Verification items for this drawing (mm, ordinates from the low corner). A direction names the side the tool comes from. Coordinates: 2 decimals unless noted, no trailing zeros. Order: outer loops, then holes, each group sorted by start corner. A loop starts at its lowest first (then second) coordinate and runs counter-clockwise, first axis right, second up. Notation, with made-up numbers: M 61,47.5 L 72,47.5 A20 ccw 72,68.5 Z; hole C 37,25.25 d10. An arc over 180 degrees is marked long. Write item = value, one per line.
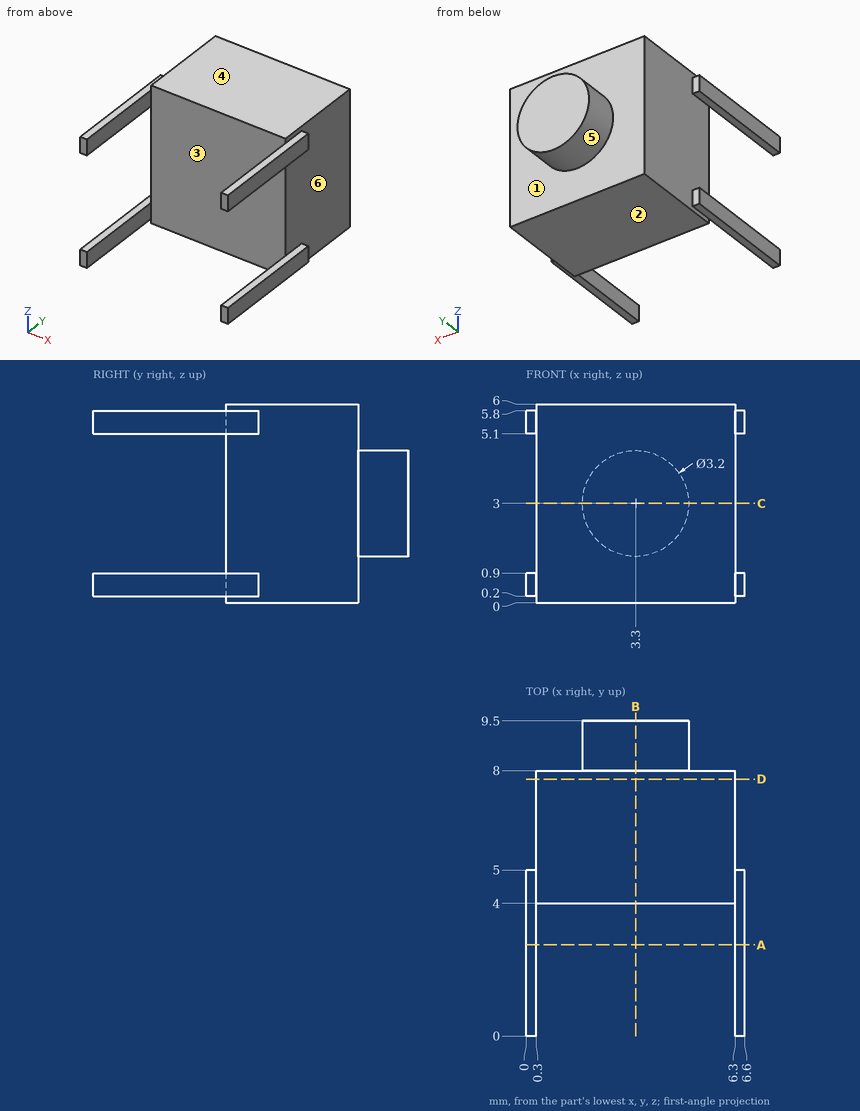
Item 1: Sectioned sample at D-D, the plane y = 7.75. Enter the section's corners in (x, z).
Report:
outline = M 0.3,0 L 6.3,0 L 6.3,6 L 0.3,6 Z
Item 2: Scan lines: L1, parallel to Y at x = 0.5, z = 0.7; L2, parallel to Y at x = 2.5, z = 1.85; L3, parallel to X at y = 6, z = 2.05. Record each from-to range of solid material in increasing order. Write a range as from..to.
Report:
L1 = 4..8
L2 = 4..9.5
L3 = 0.3..6.3
Item 3: Sectioned sample at C-C, the plane z = 3. Enter the section's corners in (x, y), then the cut area to 3 significant figures.
Report:
outline = M 0.3,4 L 6.3,4 L 6.3,8 L 4.9,8 L 4.9,9.5 L 1.7,9.5 L 1.7,8 L 0.3,8 Z
area = 28.8 mm^2
Item 4: Gauge pin test, flat ends, axial feed: pin 1 (3 mm diameter, centred on y = 6, z = 3, fed in from +X); pin 2 (3 mm diameter, centred on x = 3.5, z = 3, fed in from -Y). Record the tip position at first contact, or that the pin passes through.
Report:
pin_1 = 6.3
pin_2 = 4
Item 5: Sectioned sample at A-A, the plane y = 2.75. Enter the section's corners in (x, z), then the cut area to 3 significant figures.
Report:
outline = M 0,0.2 L 0.3,0.2 L 0.3,0.9 L 0,0.9 Z; M 0,5.1 L 0.3,5.1 L 0.3,5.8 L 0,5.8 Z; M 6.3,0.2 L 6.6,0.2 L 6.6,0.9 L 6.3,0.9 Z; M 6.3,5.1 L 6.6,5.1 L 6.6,5.8 L 6.3,5.8 Z
area = 0.840 mm^2
Item 6: Tool access check on the marked faces 1, 2 and 3. Record the directions out of +Z, -Z, +X, -X, +Y, -Y that give a thin tool (end or side, any length) a straight path to the whole face; none if there is none.
Report:
face_1 = +Y
face_2 = -Z, +X, -X, +Y, -Y
face_3 = +Z, -Z, -Y
Item 7: Release check for a two-part mould opening along Z. For the marked faces 4, 5 and 6 record: pulls with the +Z half, pulls with the -Z half, needs draft (parallel to the pull), parting line crosses it, or undercut.
Report:
face_4 = pulls with the +Z half
face_5 = parting line crosses it
face_6 = undercut
Item 8: Sectioned sample at B-B, the plane x = 3.3. Enter the section's corners in (y, z).
Report:
outline = M 4,0 L 8,0 L 8,1.4 L 9.5,1.4 L 9.5,4.6 L 8,4.6 L 8,6 L 4,6 Z
